Design review of the part shown in the three views and the two pictorial views. Dimensions are in mm from the part's minimum x, y and z. A direction names the side the tool comes from. Round coordinates to 2 decimals unless told otherwise and drop trailing zeros. Loops run counter-clockwise (first coordinate to the right, second up) from the corner with the lowest first, then second, coordinate; pieces in that order, holes last.
1. Draft analysis for pull direction X (two halves, no side actions). For the marked faces 6, 7 and 8, state which applies: released by +X, released by -X, zero draft, split by the parting line, or undercut.
2. Consider section D-D on y = 1.5. State the section outline as (x, z) points.
3. Consider section C-C on x = 1.5. State the section outline as (y, z) points, then the cut area to 3 significant figures.
4. Consider section B-B on z = 7.5. State the section outline as (x, y) points, then the cut area to 3 significant figures.
5. To check wall thickness, follow line 1 along Y through (x, z) = (1, 17); line 2 along Z through (x, y) = (9.25, 2.25); line 3 along Z through (x, y) = (13.75, 4.2). State the ranges of each line that lie inside material, in increasing order.
6. Consider section A-A on y = 3.8. State the section outline as (x, z) points, then the cut area to 3 significant figures.
7. Clearance check with flat-ended pins moving along their axes: pin 1 Ø1.6 at (y, z) = (2, 28.5) entering from -X; pin 2 Ø5 at (x, z) = (9.5, 18.5) entering from +Y; pin 3 Ø3 at (x, y) = (13.5, 3) entering from -Z. State where each tip first meets the part, or that it passes through.
8. Tool access review of the marked faces 1, 2, 3, 4 and 5: name each direction out of +Z, -Z, +X, -X, +Y, -Y from which nothing blocks a thin tool from reaching the whole face with its end or side.
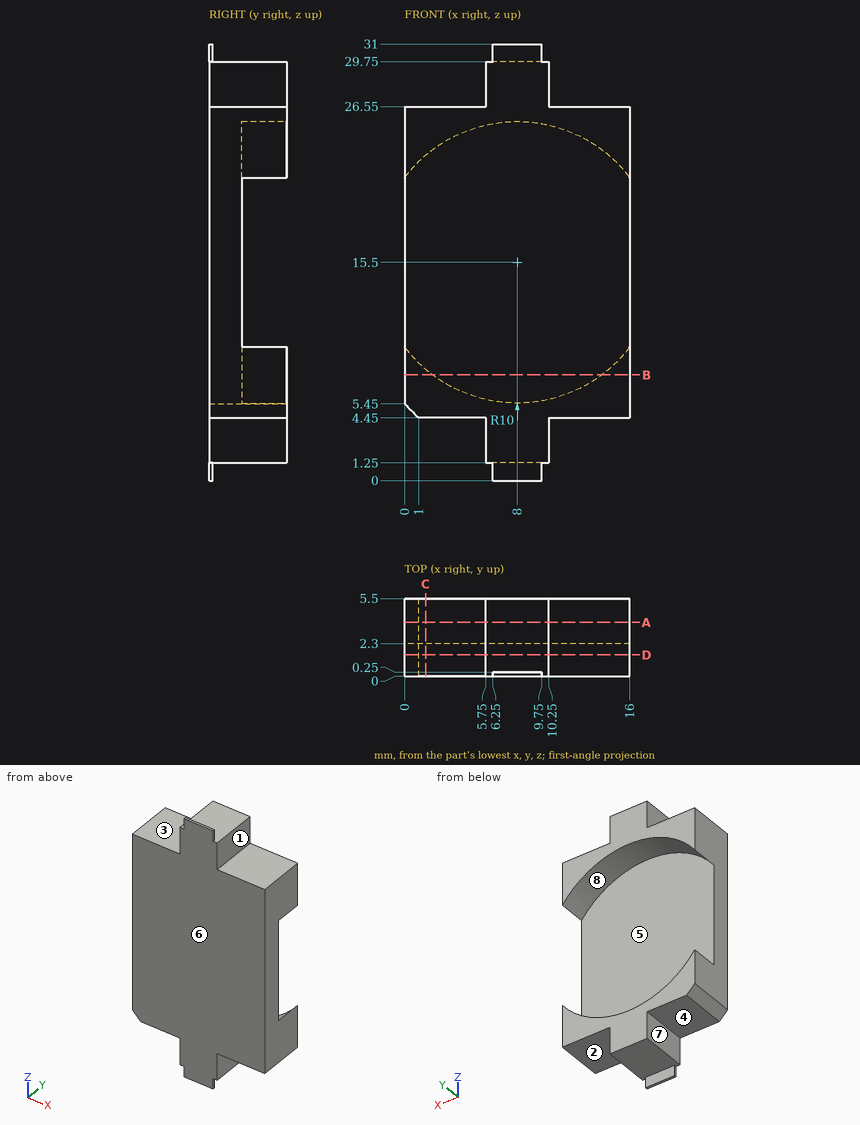
Resolved:
1. face 6: zero draft
1. face 7: released by -X
1. face 8: undercut
2. outline: (0, 5.45) - (1, 4.45) - (5.75, 4.45) - (5.75, 1.25) - (10.25, 1.25) - (10.25, 4.45) - (16, 4.45) - (16, 26.55) - (10.25, 26.55) - (10.25, 29.75) - (5.75, 29.75) - (5.75, 26.55) - (0, 26.55) - close
3. outline: (0, 4.45) - (5.5, 4.45) - (5.5, 7.9) - (2.3, 7.9) - (2.3, 23.1) - (5.5, 23.1) - (5.5, 26.55) - (0, 26.55) - close
3. area: 72.9 mm2
4. outline: (0, 0) - (16, 0) - (16, 5.5) - (14, 5.5) - (14, 2.3) - (2, 2.3) - (2, 5.5) - (0, 5.5) - close
4. area: 49.6 mm2
5. line 1: y = 0 to 2.3
5. line 2: z = 1.25 to 29.75
5. line 3: z = 4.45 to 7.32, 23.68 to 26.55
6. outline: (0, 5.45) - (1, 4.45) - (5.75, 4.45) - (5.75, 1.25) - (10.25, 1.25) - (10.25, 4.45) - (16, 4.45) - (16, 9.5) arc R10 cw to (0, 9.5) - close; (0, 21.5) arc R10 cw to (16, 21.5) - (16, 26.55) - (10.25, 26.55) - (10.25, 29.75) - (5.75, 29.75) - (5.75, 26.55) - (0, 26.55) - close
6. area: 100 mm2
7. pin 1: stops at x = 5.75
7. pin 2: stops at y = 2.3
7. pin 3: stops at z = 4.45
8. face 1: +Z, +X, +Y, -Y
8. face 2: -Z, +X, +Y, -Y
8. face 3: +Z, -X, +Y, -Y
8. face 4: -Z, -X, +Y, -Y
8. face 5: +Y
